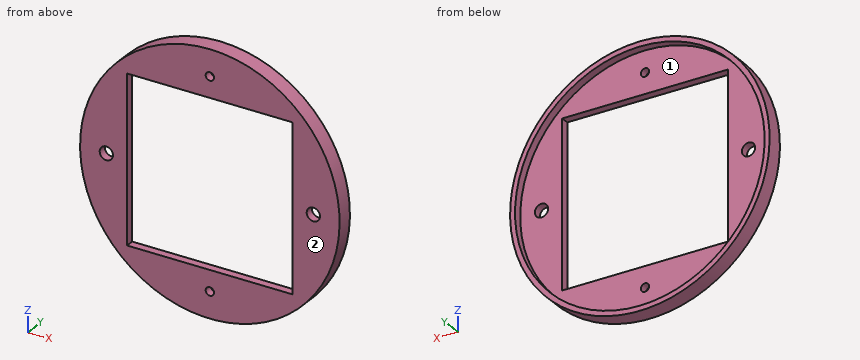
from build123d import *

# Parameters (mm, degrees)
SKETCH1_R           = 78.35
SKETCH1_R_2         = 4
SKETCH1_R_3         = 2.5
SKETCH1_W           = 100
SKETCH1_H           = 100
BOSS_EXTRUDE1_DEPTH = 5
SKETCH2_R           = 78.35
SKETCH2_R_2         = 75.35
BOSS_EXTRUDE2_DEPTH = 5


with BuildPart() as part:
    # Sketch1 → Boss-Extrude1 (new body)
    with BuildSketch(Plane(origin=(0, 0, 0), x_dir=(1, 0, 0), z_dir=(0, 1, 0))):
        with Locations(Location((0, 0, 0), (0, 0, 270))):
            Circle(SKETCH1_R)
        with Locations(Location((-62.5, 0, 0), (0, 0, 270))):
            Circle(SKETCH1_R_2, mode=Mode.SUBTRACT)
        with Locations(Location((62.5, 0, 0), (0, 0, 270))):
            Circle(SKETCH1_R_2, mode=Mode.SUBTRACT)
        with Locations(Location((0, 62.5, 0), (0, 0, 270))):
            Circle(SKETCH1_R_3, mode=Mode.SUBTRACT)
        with Locations(Location((0, -62.5, 0), (0, 0, 270))):
            Circle(SKETCH1_R_3, mode=Mode.SUBTRACT)
        Rectangle(SKETCH1_W, SKETCH1_H, mode=Mode.SUBTRACT)
    extrude(amount=BOSS_EXTRUDE1_DEPTH)

    # Sketch2 → Boss-Extrude2 (add)
    with BuildSketch(Plane(origin=(0, 5, 0), x_dir=(1, 0, 0), z_dir=(0, 1, 0))):
        with Locations(Location((0, 0, 0), (0, 0, 270))):
            Circle(SKETCH2_R)
        with Locations(Location((0, 0, 0), (0, 0, 270))):
            Circle(SKETCH2_R_2, mode=Mode.SUBTRACT)
    extrude(amount=BOSS_EXTRUDE2_DEPTH)


solid = part.part
For this review, take the finished solid that the model builds, in its own axes (mm). Face numbers are marked on the shaded views. Coordinates: 2 decimals unless noted, no trailing zeros. Loops run counter-clockwise (first coordinate to the right, second up) from the corner with the lowest first, then second, coordinate; pieces in that order, holes last. Notation, with made-up numbers: (54, 56.25) - (113, 56.25) arc R26 cw to (113, 87.25) - close; hole circle Ø7 at (8, -22). An arc over 180 degrees is marked (long way). Return JSON: item names as keys, results as strings.
Item 1: Take a section at D-D (x = -40). Give the boundary of the cut face in (y, z).
Determined:
{"outline": "(0, -67.37) - (10, -67.37) - (10, -63.86) - (5, -63.86) - (5, -50) - (0, -50) - close; (0, 50) - (5, 50) - (5, 63.86) - (10, 63.86) - (10, 67.37) - (0, 67.37) - close"}
Item 2: Take a section at B-B (z = 0). Give the boundary of the cut face in (x, y).
Determined:
{"outline": "(-78.35, 0) - (-66.5, 0) - (-66.5, 5) - (-75.35, 5) - (-75.35, 10) - (-78.35, 10) - close; (-58.5, 0) - (-50, 0) - (-50, 5) - (-58.5, 5) - close; (50, 0) - (58.5, 0) - (58.5, 5) - (50, 5) - close; (66.5, 0) - (78.35, 0) - (78.35, 10) - (75.35, 10) - (75.35, 5) - (66.5, 5) - close"}
Item 3: For line 1 (X direction, y = 2.9, z = 0); line 2 (X direction, y = 7.5, z = 0); line 3 (Z direction, x = -2, y = 6), list the stretches that pass through material, from the lowest coordinate up.
Determined:
{"line 1": "x = -78.35 to -66.5, -58.5 to -50, 50 to 58.5, 66.5 to 78.35", "line 2": "x = -78.35 to -75.35, 75.35 to 78.35", "line 3": "z = -78.32 to -75.32, 75.32 to 78.32"}
Item 4: Mouldability with a two-part tool opening along X and no side actions: class the marked faces 1 and 2 as pulls with the +X half, pulls with the -X half, needs draft (parallel to the pull), parting line crosses it, or undercut.
Determined:
{"face 1": "undercut", "face 2": "needs draft"}
Item 5: Insertion check: pin 1 (4 mm diameter, centred on x = 23.5, y = 8.5, fed in from +Z); pin 2 (5.5 mm diameter, centred on y = 3, z = 24.5, fed in from +X); pin 3 (10.5 mm diameter, centred on x = -62.5, z = 0, fed in from +Y); pin 4 (6.5 mm diameter, centred on x = 62.5, z = 0, fed in from +Y). Each pin has a flat end and moves straight along its axis. Give the tip position at first contact, or say it passes through.
Determined:
{"pin 1": "stops at z = 75.34", "pin 2": "stops at x = 75.27", "pin 3": "stops at y = 5", "pin 4": "passes through"}
Item 6: Take a section at C-C (z = 62.5). Give the boundary of the cut face in (x, y).
Determined:
{"outline": "(-47.25, 0) - (-2.5, 0) - (-2.5, 5) - (-42.09, 5) - (-42.09, 10) - (-47.25, 10) - close; (2.5, 0) - (47.25, 0) - (47.25, 10) - (42.09, 10) - (42.09, 5) - (2.5, 5) - close"}
Item 7: Take a section at A-A (x = 0). Give the boundary of the cut face in (y, z), then the cut area to 4 significant figures.
Determined:
{"outline": "(0, -78.35) - (10, -78.35) - (10, -75.35) - (5, -75.35) - (5, -65) - (0, -65) - close; (0, -60) - (5, -60) - (5, -50) - (0, -50) - close; (0, 50) - (5, 50) - (5, 60) - (0, 60) - close; (0, 65) - (5, 65) - (5, 75.35) - (10, 75.35) - (10, 78.35) - (0, 78.35) - close", "area": "263.5 mm2"}
